Work out the finished part from the listing and answer in its coordinate system (mm). Give positions to 0.01 mm unless a question says otherwise; leave off trailing zeros. Order: outer loops, then holes, each group sorted by start corner. A loop starts at its lowest first (then second) coordinate and runs counter-clockwise, first axis right, second up.
```python
from build123d import *

# Parameters (mm, degrees)
SKETCH1_R               = 2.38125
BOSS_EXTRUDE1_DEPTH     = 1.5875
SKETCH2_R               = 3.175
BOSS_EXTRUDE2_DEPTH     = 1.5875
SKETCH3_R               = 2.38125
BOSS_EXTRUDE3_DEPTH     = 19.05
SKETCH4_R               = 3.175
BOSS_EXTRUDE4_DEPTH     = 1.5875
SKETCH5_R               = 2.38125
BOSS_EXTRUDE5_DEPTH     = 1.5875
SKETCH6_R               = 2.38125
CUT_EXTRUDE1_DEPTH      = 28.662025878
SKETCH7_W               = 40.69090725
SKETCH7_H               = 20.005301762
CUT_EXTRUDE2_DEPTH      = 26.381492779
CUT_EXTRUDE3_DEPTH      = 19.487872394
CUT_EXTRUDE3_DEPTH_BACK = 19.487872394
SKETCH8_R               = 2.38125


with BuildPart() as part:
    # Sketch1 → Boss-Extrude1 (new body)
    with BuildSketch(Plane(origin=(0, 0, 0), x_dir=(1, 0, 0), z_dir=(0, 1, 0))):
        with BuildLine():
            Line((9.398005644, 4.762076723), (-6.35, 4.7625))
            ThreePointArc((-6.35, 4.7625), (-11.020584629, 0.931152767), (-8.176363381, -4.398386414))
            ThreePointArc((-8.176363381, -4.398386414), (-5.292234705, -6.221263486), (-3.181508348, -8.901918869))
            ThreePointArc((-3.181508348, -8.901918869), (1.849687492, -11.693035316), (6.504625866, -8.311495529))
            ThreePointArc((6.504625866, -8.311495529), (8.146827792, -5.96033805), (10.67447942, -4.60544104))
            ThreePointArc((10.67447942, -4.60544104), (14.180390361, 0.643024113), (9.398005644, 4.762076723))
        make_face()
        with Locations(Location((-6.35, 0, 0), (0, 0, 270))):
            Circle(SKETCH1_R, mode=Mode.SUBTRACT)
        with Locations(Location((9.4615, 0, 0), (0, 0, 270))):
            Circle(SKETCH1_R, mode=Mode.SUBTRACT)
        with Locations(Location((1.524, -6.35, 0), (0, 0, 270))):
            Circle(SKETCH1_R, mode=Mode.SUBTRACT)
    extrude(amount=BOSS_EXTRUDE1_DEPTH)

    # Sketch2 → Boss-Extrude2 (add)
    with BuildSketch(Plane.XZ):
        with Locations(Location((1.524, 6.35, 0), (0, 0, 90))):
            Circle(SKETCH2_R)
    extrude(amount=BOSS_EXTRUDE2_DEPTH)

    # Sketch3 → Boss-Extrude3 (add)
    with BuildSketch(Plane(origin=(0, 0, 0), x_dir=(1, 0, 0), z_dir=(0, 1, 0))):
        with Locations(Location((1.524, -6.35, 0), (0, 0, 90))):
            Circle(SKETCH3_R)
    extrude(amount=BOSS_EXTRUDE3_DEPTH)

    # Sketch4 → Boss-Extrude4 (add)
    with BuildSketch(Plane(origin=(0, 19.05, 0), x_dir=(1, 0, 0), z_dir=(0, 1, 0))):
        with Locations(Location((1.524, -6.35, 0), (0, 0, 270))):
            Circle(SKETCH4_R)
    extrude(amount=-BOSS_EXTRUDE4_DEPTH)

    # Sketch6 → Cut-Extrude1 (cut, through all)
    with BuildSketch(Plane(origin=(0, 19.05, 0), x_dir=(1, 0, 0), z_dir=(0, 1, 0))):
        with Locations(Location((1.524, -6.35, 0), (0, 0, 90))):
            Circle(SKETCH6_R)
    extrude(amount=-CUT_EXTRUDE1_DEPTH, mode=Mode.SUBTRACT)


with BuildPart() as body_2:
    # Sketch5 → Boss-Extrude5 (new body)
    with BuildSketch(Plane.XZ.offset(-17.4625)):
        with BuildLine():
            ThreePointArc((-8.176363381, 4.398386414), (-11.020584629, -0.931152767), (-6.35, -4.7625))
            Line((-6.35, -4.7625), (9.4615, -4.7625))
            ThreePointArc((9.4615, -4.7625), (14.184572051, -0.611552653), (10.67447942, 4.60544104))
            ThreePointArc((10.67447942, 4.60544104), (8.146827792, 5.96033805), (6.504625866, 8.311495529))
            ThreePointArc((6.504625866, 8.311495529), (1.849687492, 11.693035316), (-3.181508348, 8.901918869))
            ThreePointArc((-3.181508348, 8.901918869), (-5.292234705, 6.221263486), (-8.176363381, 4.398386414))
        make_face()
        with Locations(Location((-6.35, 0, 0), (0, 0, 270))):
            Circle(SKETCH5_R, mode=Mode.SUBTRACT)
        with Locations(Location((9.4615, 0, 0), (0, 0, 270))):
            Circle(SKETCH5_R, mode=Mode.SUBTRACT)
        with Locations(Location((1.524, 6.35, 0), (0, 0, 270))):
            Circle(SKETCH5_R, mode=Mode.SUBTRACT)
    extrude(amount=BOSS_EXTRUDE5_DEPTH)


with BuildPart() as cut_extrude1_piece_1:
    # of the separate pieces the step leaves, piece 1, a body of its own (cut_extrude1_pieces)
    add(part.part.solids().sort_by_distance((9.398005644, 0, -4.762076723))[0])

    # Sketch7 → Cut-Extrude2 (cut, through all)
    with BuildSketch(Plane(origin=(0, 1.5875, 0), x_dir=(1, 0, 0), z_dir=(0, 1, 0))):
        with Locations((0.04887425, -4.128782639)):
            Rectangle(SKETCH7_W, SKETCH7_H)
    extrude(amount=-CUT_EXTRUDE2_DEPTH, mode=Mode.SUBTRACT)


with BuildPart() as cut_extrude1_piece_2:
    # of the separate pieces the step leaves, piece 2, a body of its own (cut_extrude1_pieces)
    add(part.part.solids().sort_by_distance((1.524, 17.4625, 9.525))[0])


with BuildPart() as cut_extrude3_tool:
    # Sketch8 → Cut-Extrude3 (new, two sides: drawn at the far end of the back side and taken through both)
    # profile 1 of 2: a face of its own
    with BuildSketch(Plane(origin=(0, 17.4625, 0), x_dir=(1, 0, 0), z_dir=(0, 1, 0)).offset(-CUT_EXTRUDE3_DEPTH_BACK)):
        with BuildLine():
            Line((14.224, 0), (11.84275, 0))
            ThreePointArc((11.84275, 0), (9.4615, -2.38125), (7.08025, 0))
            Line((7.08025, 0), (-3.96875, 0))
            ThreePointArc((-3.96875, 0), (-6.35, -2.38125), (-8.73125, 0))
            Line((-8.73125, 0), (-11.1125, 0))
            ThreePointArc((-11.1125, 0), (-10.311026499, -2.644177627), (-8.176363381, -4.398386414))
            ThreePointArc((-8.176363381, -4.398386414), (-5.292234705, -6.221263486), (-3.181508348, -8.901918869))
            ThreePointArc((-3.181508348, -8.901918869), (1.849687492, -11.693035316), (6.504625866, -8.311495529))
            ThreePointArc((6.504625866, -8.311495529), (8.146827792, -5.96033805), (10.67447942, -4.60544104))
            ThreePointArc((10.67447942, -4.60544104), (13.233649304, -2.907283248), (14.224, 0))
        make_face()
        with Locations((1.524, -6.35)):
            Circle(SKETCH8_R, mode=Mode.SUBTRACT)
    # profile 2 of 2: a face of its own
    with BuildSketch(Plane(origin=(0, 17.4625, 0), x_dir=(1, 0, 0), z_dir=(0, 1, 0)).offset(-CUT_EXTRUDE3_DEPTH_BACK)):
        with Locations((1.524, -6.35)):
            Circle(SKETCH8_R)
    extrude(amount=CUT_EXTRUDE3_DEPTH + CUT_EXTRUDE3_DEPTH_BACK)


with BuildPart() as body_2_1:
    add(body_2.part)

    # Cut-Extrude3: cut by cut_extrude3_tool
    add(cut_extrude3_tool.part, mode=Mode.SUBTRACT)


with BuildPart() as cut_extrude1_piece_2_1:
    add(cut_extrude1_piece_2.part)

    # Cut-Extrude3: cut by cut_extrude3_tool
    add(cut_extrude3_tool.part, mode=Mode.SUBTRACT)


solid = body_2_1.part
```
1. The part is cut by section A-A (z = -0.4). Write down the section's boundary in (x, y) (1 decimal).
Findings below:
outline: (-11.1, 15.9) - (-8.7, 15.9) - (-8.7, 17.5) - (-11.1, 17.5) - close; (-4, 15.9) - (7.1, 15.9) - (7.1, 17.5) - (-4, 17.5) - close; (11.8, 15.9) - (14.2, 15.9) - (14.2, 17.5) - (11.8, 17.5) - close
2. Straight lines are drawn through the part: probe 1 along X at (y, z) = (17, -0.45); probe 2 along X at (y, z) = (16.7, -2.1); probe 3 along Z at (x, y) = (-6.25, 16.2). For each, find the intervals that lie inside material, in ascending order.
Findings below:
probe 1: x = -11.09 to -8.69, -4.01 to 7.12, 11.8 to 14.2
probe 2: x = -10.62 to -7.47, -5.23 to 8.34, 10.58 to 13.74
probe 3: z = -4.76 to -2.38
3. The part is cut by section D-D (z = -3.85). Write down the section's boundary in (x, y) (1 decimal).
Findings below:
outline: (-9.2, 15.9) - (12.3, 15.9) - (12.3, 17.5) - (-9.2, 17.5) - close
4. The mould has two halves that part along X. Classify faces 1 (the face through (-6.4, 16.68, -2.38)), 2 (the face through (1, 17, -4.762)), 3 (the face through (-9.754, 16.68, -3.33)), 4 (the face through (12.792, 16.68, -3.404)): pulls with the +X half, pulls with the -X half, needs draft (parallel to the pull), parting line crosses it, or undercut.
Findings below:
face 1: undercut
face 2: needs draft
face 3: pulls with the -X half
face 4: pulls with the +X half
5. The part is cut by section C-C (x = -6). Write down the section's boundary in (y, z) (1 decimal), then the cut area to 3 significant figures.
Findings below:
outline: (15.9, -4.8) - (17.5, -4.8) - (17.5, -2.4) - (15.9, -2.4) - close
area: 3.82 mm2
